from build123d import *

# Parameters (mm, degrees)
F0_R     = 2.5
F1_DEPTH = 12.5


with BuildPart() as f1:
    # F0 (on Front) → F1 (new body)
    with BuildSketch(Plane.XZ):
        Polygon((30, 73.480435), (-30, 73.480435), (-60, 60), (-60, 14.888939), (-30, -73.480435), (30, -73.480435), (35.737889, -56.578646), (40.796766, -41.676988), (60, 14.888939), (60, 60), align=None)
        with Locations((-15.7, -56.578646)):
            Circle(F0_R, mode=Mode.SUBTRACT)
        with Locations((-15.7, -41.676988)):
            Circle(F0_R, mode=Mode.SUBTRACT)
        with Locations((15.7, -56.578646)):
            Circle(F0_R, mode=Mode.SUBTRACT)
        with Locations((15.7, -41.676988)):
            Circle(F0_R, mode=Mode.SUBTRACT)
        with Locations((-32.532971, 34.246657)):
            Circle(F0_R, mode=Mode.SUBTRACT)
        with Locations((-42.327315, 48.736922)):
            Circle(F0_R, mode=Mode.SUBTRACT)
        with Locations((32.53, 34.246657)):
            Circle(F0_R, mode=Mode.SUBTRACT)
        with Locations((42.33, 48.406292)):
            Circle(F0_R, mode=Mode.SUBTRACT)
    extrude(amount=F1_DEPTH)


solid = f1.part
CAD build for the part. Positions are in the model's coordinates, mm. Coordinates: 2 decimals unless noted, no trailing zeros. Order: outer loops, then holes, each group sorted by start corner. A loop starts at its lowest first (then second) coordinate and runs counter-clockwise, first axis right, second up.
Item 1: Pin check, flat tips, straight feed: pin 1 Ø3 at (x, z) = (15.7, -56.58) entering from +Y; pin 2 Ø1 at (y, z) = (-5, -51) entering from +X. Stop position of each tip, or through.
Check sheet entries:
pin 1: passes through
pin 2: stops at x = 37.8
Item 2: Band-saw the part on A-A on x = 15.7. List the corners of the cut face in (y, z), plus the area to 3 significant figures.
Check sheet entries:
outline: (-12.5, -73.48) - (0, -73.48) - (0, -59.08) - (-12.5, -59.08) - close; (-12.5, -54.08) - (0, -54.08) - (0, -44.18) - (-12.5, -44.18) - close; (-12.5, -39.18) - (0, -39.18) - (0, 73.48) - (-12.5, 73.48) - close
area: 1,710 mm2
Item 3: Band-saw the part on D-D on z = -13. List the corners of the cut face in (x, y).
Check sheet entries:
outline: (-50.53, -12.5) - (50.53, -12.5) - (50.53, 0) - (-50.53, 0) - close
Item 4: Band-saw the part on B-B on y = -3.75. Give the number of separate pieces and of enclosed holes in the cut face, plus the area to 3 significant figures.
Check sheet entries:
separate pieces: 1
enclosed holes: 8
area: 14,400 mm2
Item 5: Band-saw the part on C-C on x = 42.33. List the corners of the cut face in (y, z).
Check sheet entries:
outline: (-12.5, -37.16) - (0, -37.16) - (0, 45.91) - (-12.5, 45.91) - close; (-12.5, 50.91) - (0, 50.91) - (0, 67.94) - (-12.5, 67.94) - close
Item 6: Two-plate mould, pull along Z, no slides. Class faces 1 (the face through (-45.21, -6.16, -28.68)), 2 (the face through (15.16, -6.16, -59.02)), 3 (the face through (-60, -6, 38)): +Z half, -Z half, draft (parallel to the pull), parting line (faces both ways), or undercut.
Check sheet entries:
face 1: -Z half
face 2: undercut
face 3: draft
Item 7: Drill centre lines: L1, parallel to Z at x = -15.7, y = -7; L2, parallel to X at y = -2, z = 50; L3, parallel to X at y = -4, z = -66.5. Where is each one in solid material? Low to high.
Check sheet entries:
L1: z = -73.48 to -59.08, -54.08 to -44.18, -39.18 to 73.48
L2: x = -60 to -44.48, -40.17 to 40.4, 44.26 to 60
L3: x = -32.37 to 32.37
